Can you work these out from the model? Positions are in its coordinate system, mm. Face numbers are marked on the shaded views. Coordinates: 2 decimals unless noted, no trailing zeros. Loops run counter-clockwise (first coordinate to the right, second up) from the corner with the lowest first, then second, coordinate; pieces in that order, holes last. Notation, with made-up numbers: M 66,-39.5 L 84,-39.5 A27 ccw 84,-22.5 Z; hole C -36.75,63 d10. An arc over 180 degrees is marked long. Return JSON: item names as keys, results as strings. Group by question number.
```python
from build123d import *

# Parameters (mm, degrees)
SKETCH1_W           = 30
SKETCH1_H           = 30
SKETCH1_R           = 3
BOSS_EXTRUDE1_DEPTH = 9


with BuildPart() as part:
    # Sketch1 → Boss-Extrude1 (new body)
    with BuildSketch(Plane.YZ):
        Rectangle(SKETCH1_W, SKETCH1_H)
        with Locations(Location((6.050252532, 6.050252532, 0), (0, 0, 270))):
            Circle(SKETCH1_R, mode=Mode.SUBTRACT)
        with Locations(Location((-6.050252532, 6.050252532, 0), (0, 0, 270))):
            Circle(SKETCH1_R, mode=Mode.SUBTRACT)
        with Locations(Location((-6.050252532, -6.050252532, 0), (0, 0, 270))):
            Circle(SKETCH1_R, mode=Mode.SUBTRACT)
        with Locations(Location((6.050252532, -6.050252532, 0), (0, 0, 270))):
            Circle(SKETCH1_R, mode=Mode.SUBTRACT)
    extrude(amount=BOSS_EXTRUDE1_DEPTH)


solid = part.part
```
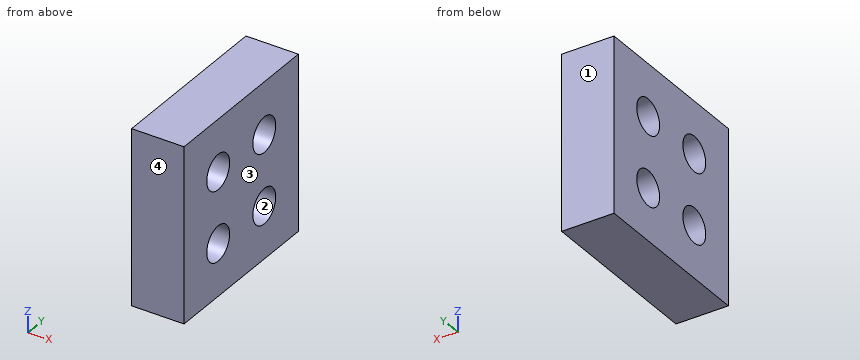
1) Suppose I cut it at B-B, the plane z = 6.25. List the corners of the cut face in (x, y) for me.
2) Suppose I cut it at A-A, the plane y = 5.5. List the corners of the cut face in (x, z) for me.
3) If I drill on line 1 (Y direction, x = 6.5, z = -6.25); line 2 (Z direction, x = 7, y = -8), over which ranges is the centre line in solid material (lowest first)? Write a range as from..to.
4) If we mould it in two halves opening along Y, with no side actions, what happens to the marked faces 1, 2, 3 and 4? For each: +Y half, -Y half, draft (parallel to the pull), parting line (faces both ways), or undercut.
5) Suppose I cut it at C-C, the plane x = 6.25. List the corners of the cut face in (y, z) for me, then the cut area to 3 significant figures.
Returned:
{
 "1": {"outline": "M 0,-15 L 9,-15 L 9,-9.04 L 0,-9.04 Z; M 0,-3.06 L 9,-3.06 L 9,3.06 L 0,3.06 Z; M 0,9.04 L 9,9.04 L 9,15 L 0,15 Z"},
 "2": {"outline": "M 0,-15 L 9,-15 L 9,-9 L 0,-9 Z; M 0,-3.1 L 9,-3.1 L 9,3.1 L 0,3.1 Z; M 0,9 L 9,9 L 9,15 L 0,15 Z"},
 "3": {"line 1": "y = -15..-9.04, -3.06..3.06, 9.04..15", "line 2": "z = -15..-8.33, -3.77..3.77, 8.33..15"},
 "4": {"face 1": "+Y half", "face 2": "undercut", "face 3": "draft", "face 4": "-Y half"},
 "5": {"outline": "M -15,-15 L 15,-15 L 15,15 L -15,15 Z; hole C -6.05,-6.05 d6; hole C -6.05,6.05 d6; hole C 6.05,-6.05 d6; hole C 6.05,6.05 d6", "area": "787 mm²"}
}
